Can you work these out from the model? Positions are in its coordinate system, mm. A direction names the side the tool comes from. Round coordinates to 2 decimals unless told otherwise and drop trailing zeros. Order: outer loops, then holes, each group sorted by start corner. A loop starts at its lowest first (then second) coordinate and runs counter-clockwise, first axis right, second up. Notation, with made-up numbers: (22, 49.25) - (47, 49.25) arc R22 cw to (47, 68.25) - close; hole circle Ø6 at (55, 6). An arc over 180 degrees is marked (long way). Write item = value, one per line.
from build123d import *

# Parameters (mm, degrees)
F0_R     = 2.2225
F0_R_2   = 1.524
F0_W     = 3.175
F0_H     = 6.35
F1_DEPTH = 3.175


# Not quite as in the source:
# - a length typed as a fraction of an inch, garbled in the dataset ("3 / 203.2 mm" for 3/8 in), is restored


with BuildPart() as f1:
    # F0 (on Top) → F1 (new body)
    with BuildSketch(Plane.XY):
        with BuildLine():
            ThreePointArc((15, 82.55), (13.1401280605, 87.0401280605), (8.65, 88.9))
            Line((8.65, 88.9), (-8.65, 88.9))
            ThreePointArc((-8.65, 88.9), (-13.1401280605, 87.0401280605), (-15, 82.55))
            Line((-15, 82.55), (-15, -82.55))
            ThreePointArc((-15, -82.55), (-13.1401280605, -87.0401280605), (-8.65, -88.9))
            Line((-8.65, -88.9), (8.65, -88.9))
            ThreePointArc((8.65, -88.9), (13.1401280605, -87.0401280605), (15, -82.55))
            Line((15, -82.55), (15, 82.55))
        make_face()
        with Locations((-5.6566, -78.197214059)):
            Circle(F0_R, mode=Mode.SUBTRACT)
        Polygon((0.75, -33.696414059), (10, -33.696414059), (10, -74.387214059), (0.75, -74.387214059), (0.75, -81.691814059), (-0.75, -81.691814059), (-0.75, -74.387214059), (-10, -74.387214059), (-10, -33.696414059), (-0.75, -33.696414059), (-0.75, -26.391814059), (0.75, -26.391814059), align=None, mode=Mode.SUBTRACT)
        with Locations((-5.6566, -29.886414059)):
            Circle(F0_R, mode=Mode.SUBTRACT)
        with Locations((5.6566, -78.197214059)):
            Circle(F0_R, mode=Mode.SUBTRACT)
        with Locations((5.6566, -29.886414059)):
            Circle(F0_R, mode=Mode.SUBTRACT)
        with Locations((0, 69.85)):
            Circle(F0_R_2, mode=Mode.SUBTRACT)
        with Locations((0, 82.55)):
            Rectangle(F0_W, F0_H, mode=Mode.SUBTRACT)
    extrude(amount=F1_DEPTH)


solid = f1.part
(1) If we section it at A-A (y = 69.85): Write out the boundary of the cut face in (x, z) (3 decimals).
Computed:
outline = (-15, 0) - (-1.524, 0) - (-1.524, 3.175) - (-15, 3.175) - close; (1.524, 0) - (15, 0) - (15, 3.175) - (1.524, 3.175) - close
(2) Will this pin go through, and if not, where does the flat tip stop? P1, Ø1, axis at x = -10, z = 2, coming from the -Y side.
Computed:
P1 = -88.84
(3) If we section it at C-C (z = 1.85): State how many separate pieces and enclosed holes the cut face has, plus the area to 3 significant figures.
Computed:
separate_pieces = 1
enclosed_holes = 7
area = 4,370 mm^2
(4) If I drill on line 1 (Y direction, x = 0, z = 1.85) (3 decimals); line 2 (X direction, y = -61, z = 2.6); line 3 (Y direction, x = 1, z = 1) (3 decimals), over which ranges is the centre line in solid material (lowest first)? Write a range as from..to.
Computed:
line_1 = -88.9..-81.692, -26.392..68.326, 71.374..79.375, 85.725..88.9
line_2 = -15..-10, 10..15
line_3 = -88.9..-74.387, -33.696..68.7, 71..79.375, 85.725..88.9
(5) Thinking about a two-plate mould opening in Y: for faces 3 (the face through (-0.75, -30, 2)), 4 (the face through (0, -88.9, 2)), 5 (the face through (-15, 1, 2)), 6 (the face through (13.19, 86.99, 1.57)), which applies, +Y half, -Y half, draft (parallel to the pull), parting line (faces both ways), or undercut?
Computed:
face_3 = undercut
face_4 = -Y half
face_5 = draft
face_6 = +Y half
(6) If we section it at B-B (x = -5.5): Write out the boundary of the cut face in (y, z) (3 decimals).
Computed:
outline = (-88.9, 0) - (-80.414, 0) - (-80.414, 3.175) - (-88.9, 3.175) - close; (-75.98, 0) - (-74.387, 0) - (-74.387, 3.175) - (-75.98, 3.175) - close; (-33.696, 0) - (-32.103, 0) - (-32.103, 3.175) - (-33.696, 3.175) - close; (-27.669, 0) - (88.9, 0) - (88.9, 3.175) - (-27.669, 3.175) - close
(7) On a 3-axis mill with a long thin cutter (end or side, diameter ignored), from which of +Z, -Z, +X, -X, +Y, -Y can I reach the whole of each face in a straight line? I mean faces 1 (the face through (-5, -33.696, 2)), 2 (the face through (-13.19, -86.99, 1.57)). Say none if no direction works.
Computed:
face_1 = +Z, -Z
face_2 = +Z, -Z, -X, -Y
